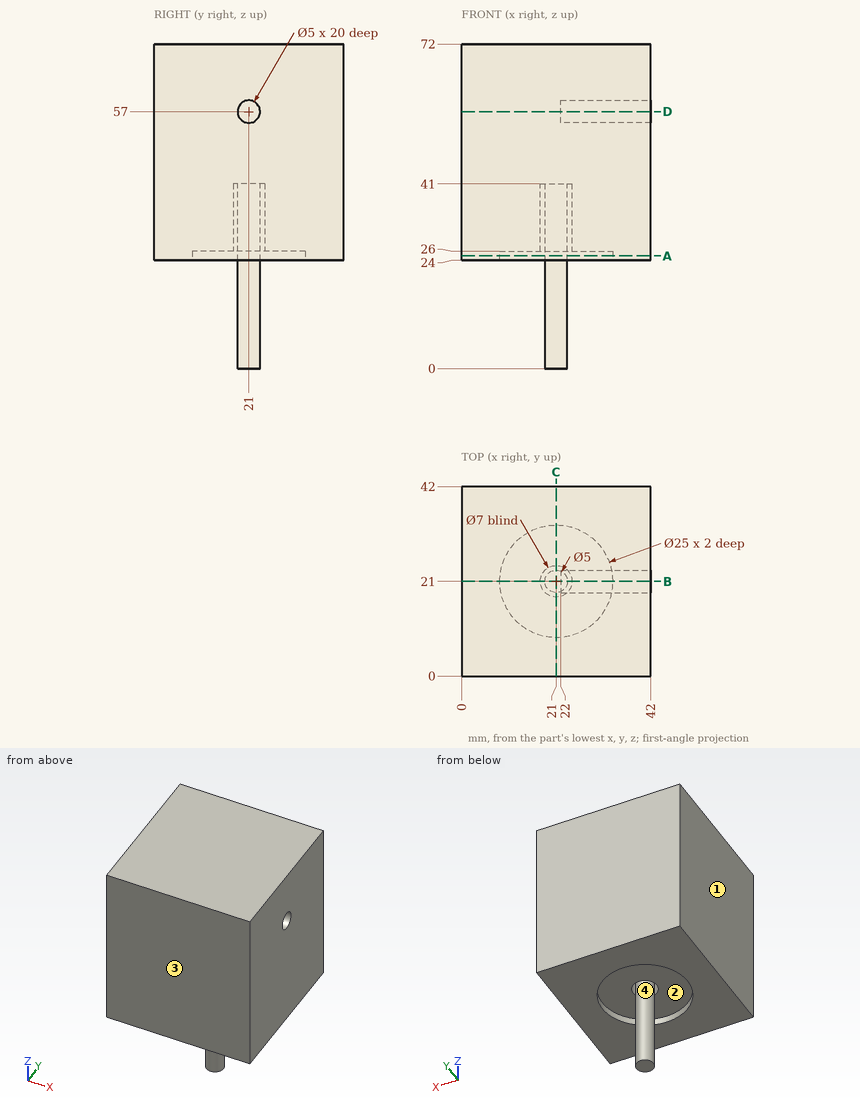
Study the drawing (mm; zero at the part's minimum x, y, z) and answer. Round coordinates to 2 decimals unless told otherwise and drop trailing zeros. Order: outer loops, then holes, each group sorted by start corner. A loop starts at its lowest first (then second) coordinate and runs counter-clockwise, first axis right, second up. Notation, with made-up numbers: (5, -31.75) - (33, -31.75) arc R12 cw to (33, -20.75) - close; hole circle Ø6 at (-15.5, -2.75). An arc over 180 degrees is marked (long way). Use one line per item in the form item = value. Start each with the question number.
(1) The part is cut by section C-C (x = 21). Give the vertices of the cut face in (y, z).
(2) The part is cut by section A-A (z = 25). Give the vertices of the cut face in (x, y).
(3) The part is cut by section B-B (y = 21). Give the vertices of the cut face in (x, z), then the cut area to 3 significant figures.
(4) Determine the mould class of the marked faces 1, 2, 3 and 4 for opening direction Y: +Y half, -Y half, draft (parallel to the pull), parting line (faces both ways), or undercut.
(5) The part is cut by section D-D (z = 57). Give the vertices of the cut face in (x, y), then the cut area to 3 significant figures.
(6) Find the intervals of material crossed by line 1 along Y through (x, z) = (21, 31); line 2 along Y through (x, z) = (21, 25); line 3 along Y through (x, z) = (37, 57), in increasing order. Write a range as from..to.
(7) Flat-ended cylindrical pins translate along their axes: pin 1 Ø4 at (y, z) = (20, 36.5) entering from -X; pin 2 Ø1.5 at (x, y) = (21, 25) entering from -Z; pin 3 Ø1.5 at (y, z) = (20, 57.5) entering from +X. Find the tip coordinate at first contact, or state that the pin passes through.
Checked values:
q1.outline = (0, 24) - (8.5, 24) - (8.5, 26) - (17.5, 26) - (17.5, 41) - (18.5, 41) - (18.5, 0) - (23.5, 0) - (23.5, 41) - (24.5, 41) - (24.5, 26) - (33.5, 26) - (33.5, 24) - (42, 24) - (42, 72) - (0, 72) - close
q2.outline = (0, 0) - (42, 0) - (42, 42) - (0, 42) - close; circle Ø5 at (21, 21); hole circle Ø25 at (21, 21)
q3.outline = (0, 24) - (8.5, 24) - (8.5, 26) - (17.5, 26) - (17.5, 41) - (18.5, 41) - (18.5, 0) - (23.5, 0) - (23.5, 41) - (24.5, 41) - (24.5, 26) - (33.5, 26) - (33.5, 24) - (42, 24) - (42, 54.5) - (22, 54.5) - (22, 59.5) - (42, 59.5) - (42, 72) - (0, 72) - close
q3.area = 1,970 mm^2
q4.face_1 = draft
q4.face_2 = undercut
q4.face_3 = -Y half
q4.face_4 = undercut
q5.outline = (0, 0) - (42, 0) - (42, 18.5) - (22, 18.5) - (22, 23.5) - (42, 23.5) - (42, 42) - (0, 42) - close
q5.area = 1,660 mm^2
q6.line_1 = 0..17.5, 18.5..23.5, 24.5..42
q6.line_2 = 0..8.5, 18.5..23.5, 33.5..42
q6.line_3 = 0..18.5, 23.5..42
q7.pin_1 = 0
q7.pin_2 = 26
q7.pin_3 = 22
